```python
from build123d import *

# Parameters (mm, degrees)
F1_DEPTH  = 25.4
F3_DEPTH  = 12.701
F5_DEPTH  = 38.101
F6_R      = 12.6897983803
F7_DEPTH  = 25.4
F8_R      = 6.35
F9_DEPTH  = 38.101
F11_DEPTH = 12.701


with BuildPart() as f1:
    # F0 (on Front) → F1 (new body)
    with BuildSketch(Plane.XZ):
        Polygon((-67.8916360141, 50.7466404207), (-67.8916360141, 47.1607576076), (-67.8916360141, 12.6466404207), (8.3083639859, 12.6466404207), (8.3083639859, 25.3466404207), (-42.4916360141, 25.3466404207), (-42.4916360141, 50.7466404207), align=None)
    extrude(amount=F1_DEPTH)

    # F2 (on face) → F3 (cut, through all)
    with BuildSketch(Plane.XY.offset(25.3466404207)):
        with BuildLine():
            ThreePointArc((1.9583639859, 0), (6.632395643, -5.6004841714), (8.3083639859, -12.7))
            Line((8.3083639859, -12.7), (8.3083639859, 0))
            Line((8.3083639859, 0), (1.9583639859, 0))
        make_face()
        with BuildLine():
            ThreePointArc((8.3083639859, -12.7), (6.632395643, -19.7995158286), (1.9583639859, -25.4))
            Line((1.9583639859, -25.4), (8.3083639859, -25.4))
            Line((8.3083639859, -25.4), (8.3083639859, -12.7))
        make_face()
    extrude(amount=-F3_DEPTH, mode=Mode.SUBTRACT)

    # F4 (on face) → F5 (cut, through all)
    with BuildSketch(Plane.XY.offset(50.7466404207)):
        with BuildLine():
            ThreePointArc((-67.8916360141, -12.7), (-64.1718921352, -3.7197438789), (-55.1916360141, 0))
            Line((-55.1916360141, 0), (-67.8916360141, 0))
            Line((-67.8916360141, 0), (-67.8916360141, -12.7))
        make_face()
        with BuildLine():
            Line((-67.8916360141, -25.4), (-55.1916360141, -25.4))
            ThreePointArc((-55.1916360141, -25.4), (-64.1718921352, -21.6802561211), (-67.8916360141, -12.7))
            Line((-67.8916360141, -12.7), (-67.8916360141, -25.4))
        make_face()
    extrude(amount=-F5_DEPTH, mode=Mode.SUBTRACT)

    # F6 (on face) → F7 (cut)
    with BuildSketch(Plane.XY.offset(50.7466404207)):
        with BuildLine():
            Line((-42.4916360141, -25.4), (-42.4916360141, 0))
            Line((-42.4916360141, 0), (-55.1916360141, 0))
            ThreePointArc((-55.1916360141, 0), (-67.8916360141, -12.7), (-55.1916360141, -25.4))
            Line((-55.1916360141, -25.4), (-42.4916360141, -25.4))
        make_face()
        with Locations((-55.1916360141, -12.7)):
            Circle(F6_R, mode=Mode.SUBTRACT)
    extrude(amount=-F7_DEPTH, mode=Mode.SUBTRACT)

    # F8 (on face) → F9 (cut, through all)
    with BuildSketch(Plane.XY.offset(50.7466404207)):
        with Locations((-55.1916360141, -12.7)):
            Circle(F8_R)
    extrude(amount=-F9_DEPTH, mode=Mode.SUBTRACT)

    # F10 (on face) → F11 (cut, through all)
    with BuildSketch(Plane.XY.offset(25.3466404207)):
        with BuildLine():
            ThreePointArc((-7.5666360141, -19.05), (-3.0765079536, -17.1901280605), (-1.2166360141, -12.7))
            ThreePointArc((-1.2166360141, -12.7), (-3.0765079536, -8.2098719395), (-7.5666360141, -6.35))
            Line((-7.5666360141, -6.35), (-7.5666360141, -19.05))
        make_face()
        with BuildLine():
            Line((-7.5666360141, -19.05), (-7.5666360141, -6.35))
            ThreePointArc((-7.5666360141, -6.35), (-13.9166360141, -12.7), (-7.5666360141, -19.05))
        make_face()
        with BuildLine():
            ThreePointArc((-7.5666360141, -19.05), (-13.9166360141, -12.7), (-7.5666360141, -6.35))
            Line((-7.5666360141, -6.35), (-32.9666360141, -6.35))
            ThreePointArc((-32.9666360141, -6.35), (-28.4765079536, -8.2098719395), (-26.6166360141, -12.7))
            ThreePointArc((-26.6166360141, -12.7), (-28.4765079536, -17.1901280605), (-32.9666360141, -19.05))
            Line((-32.9666360141, -19.05), (-7.5666360141, -19.05))
        make_face()
        with BuildLine():
            Line((-32.9666360141, -12.7), (-32.9666360141, -6.35))
            ThreePointArc((-32.9666360141, -6.35), (-39.3166360141, -12.7), (-32.9666360141, -19.05))
            Line((-32.9666360141, -19.05), (-32.9666360141, -12.7))
        make_face()
        with BuildLine():
            ThreePointArc((-26.6166360141, -12.7), (-28.4765079536, -8.2098719395), (-32.9666360141, -6.35))
            Line((-32.9666360141, -6.35), (-32.9666360141, -12.7))
            Line((-32.9666360141, -12.7), (-32.9666360141, -19.05))
            ThreePointArc((-32.9666360141, -19.05), (-28.4765079536, -17.1901280605), (-26.6166360141, -12.7))
        make_face()
    extrude(amount=-F11_DEPTH, mode=Mode.SUBTRACT)


solid = f1.part
```
Source: CAD feature listing. Evaluate the final solid. Frame: model axes, mm. A direction names the side the tool comes from. Coordinates: 2 decimals unless noted, no trailing zeros. Loops run counter-clockwise (first coordinate to the right, second up) from the corner with the lowest first, then second, coordinate; pieces in that order, holes last. Notation, with made-up numbers: M -23,29 L 30,29 A22 ccw 30,52 Z; hole C 82.5,31.25 d8. An arc over 180 degrees is marked long. Put each result on its own line as item: value. Start each with the question number.
1) Cut plane D-D on z = 40. Return the cut outline in (x, y).
2) Cut plane C-C on y = -13.5. Give the number of separate pieces and of enclosed holes in the cut face, then the cut area to 3 significant figures.
3) Pull-direction query (Y, two-part tool) for faces 4 (the face through (-49, -15, 50.747)), 5 (the face through (-27, 0, 19)), 6 (the face through (-20, -6.35, 19)); classes: pulls with the +Y half, pulls with the -Y half, needs draft (parallel to the pull), parting line crosses it, or undercut.
4) Contact query for flat-ended pins moving along their axis: pin 1 Ø1 at (y, z) = (-9, 29) entering from -X; pin 2 Ø2 at (y, z) = (-14.5, 34) entering from -X; pin 3 Ø1.5 at (x, z) = (-49, 32.5) entering from +Y; pin 4 Ø6 at (x, y) = (-56.5, -12) entering from -Z. Output: stop coordinate, or through.
5) Ray query, L1, parallel to X at y = -12, z = 20.5; L2, parallel to Z at x = -13.5, y = -5.25; L3, parallel to X at y = -15.75, z = 34. Return the intervals inside material, ascending. Write a range as from..to.
6) Reachability of faces 1 (the face through (-43.47, -17.56, 38.22)), 2 (the face through (-39.315, -12.56, 19.086)), 3 (the face through (-39, -10, 12.647)) from +Z, -Z, +X, -X, +Y, -Y: full face, straight path, thin tool, end or side. Return the list, or none.
7) Cut plane A-A on z = 16.5. Return the cut outline in (x, y) (3 decimals), then the cut area to 3 significant figures.
The answers:
1. outline: C -55.19,-12.7 d25.38; hole C -55.19,-12.7 d12.7
2. separate pieces: 3
2. enclosed holes: 0
2. area: 648 mm²
3. face 4: needs draft
3. face 5: pulls with the +Y half
3. face 6: undercut
4. pin 1: stops at x = -67.47
4. pin 2: stops at x = -67.86
4. pin 3: stops at y = -1.24
4. pin 4: passes through
5. L1: x = -67.87..-61.5, -48.88..-39.28, -1.26..8.29
5. L2: z = 12.65..25.35
5. L3: x = -67.51..-60.76, -49.62..-42.87
6. face 1: +Z
6. face 2: +Z, -Z
6. face 3: -Z, +X, -X, +Y, -Y
7. outline: M -55.192,-25.4 L 1.958,-25.4 A15.875 ccw 1.958,0 L -55.192,0 A12.7 ccw Z; hole C -55.192,-12.7 d12.7; hole M -32.967,-19.05 L -7.567,-19.05 A6.35 ccw -7.567,-6.35 L -32.967,-6.35 A6.35 ccw Z
7. area: 1,240 mm²
